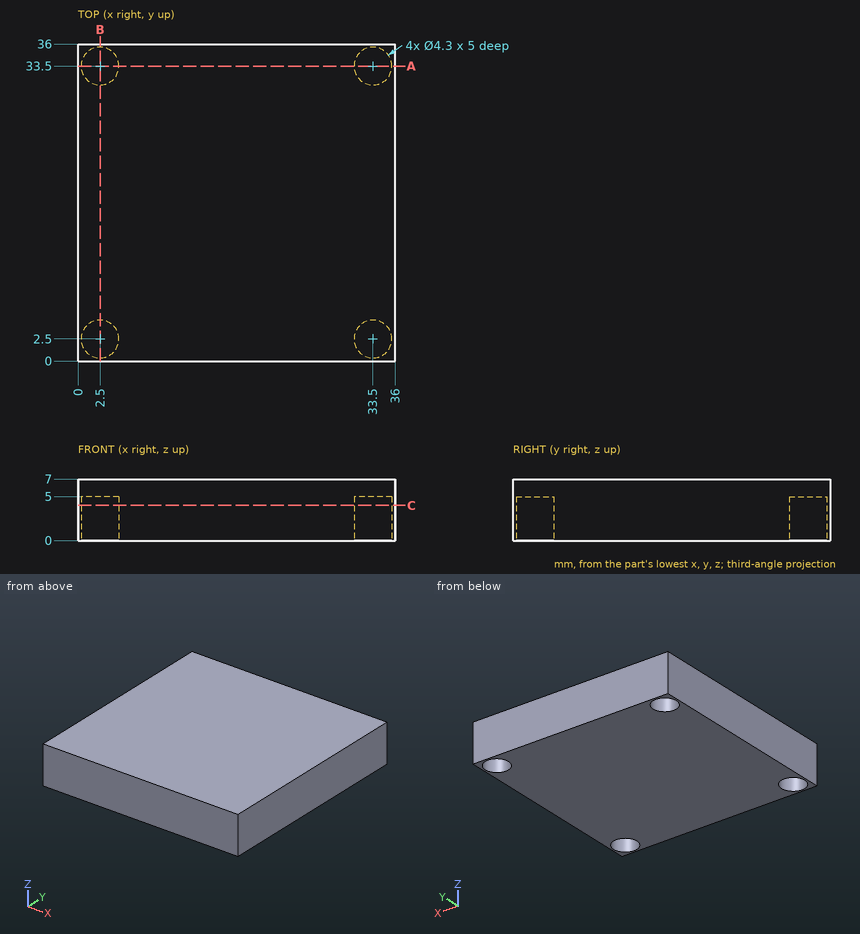
Could you check a few things on this drawing? It's one solid part, dimensions in mm from its lowest x, y, z. Give positions to 0.01 mm unless a question says otherwise; leave off trailing zeros. Write each loop counter-clockwise with the first axis right and the second up, starting at its lowest first coordinate (ties: lowest second). Pieces come first, ordered by that corner, then holes. Notation, with made-up numbers: (64.25, 74.25) -> (92.25, 74.25) arc R9 cw to (92.25, 91.25) -> close; hole circle Ø10 at (82.5, -18). An arc over 180 degrees is marked (long way). Answer as CSV lines item,"result". Start each with the question number.
(1) If we section it at C-C, the plane z = 4: Write out the boundary of the cut face in (x, y).
(2) I'm going to push a flat-ended pin straight in: pin 1 Ø1.3 at (x, y) = (34.5, 1.5) entering from -Z. Where does the tip first touch, or does it pass through?
(3) If we section it at A-A, the plane y = 33.5: Write out the boundary of the cut face in (x, z), and give its area (3 significant figures).
(4) Please list where this line runs through material, in increasing order: line 1 (Y direction, x = 2.5, z = 1.4).
Answer list:
1,outline,"(0, 0) -> (36, 0) -> (36, 36) -> (0, 36) -> close; hole circle Ø4.3 at (2.5, 2.5); hole circle Ø4.3 at (2.5, 33.5); hole circle Ø4.3 at (33.5, 2.5); hole circle Ø4.3 at (33.5, 33.5)"
2,pin 1,"z = 5"
3,outline,"(0, 0) -> (0.35, 0) -> (0.35, 5) -> (4.65, 5) -> (4.65, 0) -> (31.35, 0) -> (31.35, 5) -> (35.65, 5) -> (35.65, 0) -> (36, 0) -> (36, 7) -> (0, 7) -> close"
3,area,"209 mm^2"
4,line 1,"0 to 0.35, 4.65 to 31.35, 35.65 to 36"
